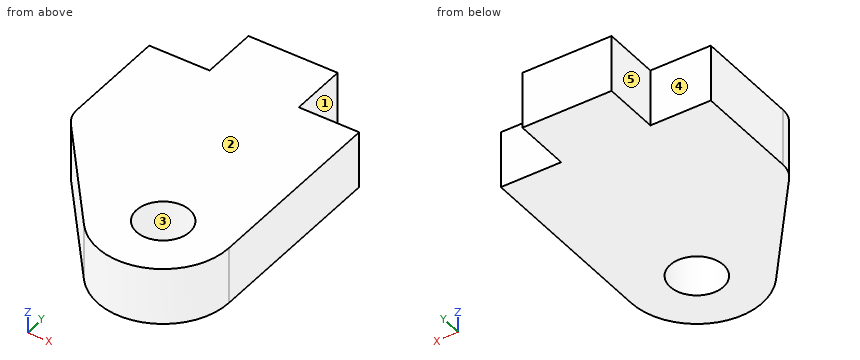
from build123d import *

# Parameters (mm, degrees)
SKETCH1_R           = 1.4859
BOSS_EXTRUDE1_DEPTH = 3.175


with BuildPart() as part:
    # Sketch1 → Boss-Extrude1 (new body)
    with BuildSketch(Plane.XY):
        with BuildLine():
            Line((-5.476150442, -1.381790583), (-0.66088404, -7.376813067))
            ThreePointArc((-0.66088404, -7.376813067), (3.40481365, -8.536580023), (5.84835, -5.08635))
            Line((5.84835, -5.08635), (5.84835, 5.56895))
            Line((5.84835, 5.56895), (2.48285, 5.56895))
            Line((2.48285, 5.56895), (2.48285, 8.74395))
            Line((2.48285, 8.74395), (-2.48285, 8.74395))
            Line((-2.48285, 8.74395), (-2.48285, 5.56895))
            Line((-2.48285, 5.56895), (-5.84835, 5.56895))
            Line((-5.84835, 5.56895), (-5.84835, -0.324042014))
            ThreePointArc((-5.84835, -0.324042014), (-5.752585393, -0.884703352), (-5.476150442, -1.381790583))
        make_face()
        with Locations((2.19075, -5.08635)):
            Circle(SKETCH1_R, mode=Mode.SUBTRACT)
    extrude(amount=BOSS_EXTRUDE1_DEPTH)


solid = part.part
Design review of the part built by this model. Coordinates are the model's own, in mm. Face numbers are marked on the shaded views. A direction names the side the tool comes from. Coordinates: 2 decimals unless noted, no trailing zeros. Order: outer loops, then holes, each group sorted by start corner. A loop starts at its lowest first (then second) coordinate and runs counter-clockwise, first axis right, second up.
Item 1: For line 1 (X direction, y = 5.75, z = 0.2); line 2 (Y direction, x = 5, z = 0.9); line 3 (X direction, y = -8, z = 1.65), list the stretches that pass through material, from the lowest coordinate up.
Item 2: Take a section at C-C, the plane y = -6.25. Write out the cut boundary in (x, z) (3 decimals).
Item 3: Take a section at A-A, the plane z = 2.7. Write out the cut boundary in (x, y), then the cut area to 3 significant figures.
Item 4: Take a section at B-B, the plane x = 1.25. Write out the cut boundary in (y, z) (3 decimals).
Item 5: For the marked faces 1 and 2, list the 3-axis set-ups (+Z, -Z, +X, -X, +Y, -Y) from which the entire face can be reached by the end or side of a thin tool; tool diameter is ignored.
Item 6: Take a section at D-D, the plane y = 7. Write out the cut boundary in (x, z) (3 decimals), then the cut area to 3 significant figures.
Item 7: For pin 1 Ø1.6 at (x, z) = (4, 1.5) entering from +Y; pin 2 Ø1.6 at (y, z) = (7.5, 1.5) entering from -X, all flat-tipped, find the tip position at first contact; note any pin that passes through.
Item 8: The part is to be moulded in two halves that separate along X. For the marked faces 3, 4 and 5, say which applies: pulls with the +X half, pulls with the -X half, needs draft (parallel to the pull), parting line crosses it, or undercut.
The answers:
1. line 1: x = -2.48 to 2.48
1. line 2: y = -7.43 to 5.57
1. line 3: x = -0.02 to 4.4
2. outline: (-1.566, 0) - (1.267, 0) - (1.267, 3.175) - (-1.566, 3.175) - close; (3.115, 0) - (5.658, 0) - (5.658, 3.175) - (3.115, 3.175) - close
3. outline: (-5.85, -0.32) arc R1.69 ccw to (-5.48, -1.38) - (-0.66, -7.38) arc R3.66 ccw to (5.85, -5.09) - (5.85, 5.57) - (2.48, 5.57) - (2.48, 8.74) - (-2.48, 8.74) - (-2.48, 5.57) - (-5.85, 5.57) - close; hole circle Ø2.97 at (2.19, -5.09)
3. area: 148 mm2
4. outline: (-8.621, 0) - (-6.237, 0) - (-6.237, 3.175) - (-8.621, 3.175) - close; (-3.936, 0) - (8.744, 0) - (8.744, 3.175) - (-3.936, 3.175) - close
5. face 1: +Z, -Z, +X, +Y
5. face 2: +Z, +X, -X, +Y, -Y
6. outline: (-2.483, 0) - (2.483, 0) - (2.483, 3.175) - (-2.483, 3.175) - close
6. area: 15.8 mm2
7. pin 1: stops at y = 5.57
7. pin 2: stops at x = -2.48
8. face 3: undercut
8. face 4: needs draft
8. face 5: pulls with the -X half
